from build123d import *

# Parameters (mm, degrees)
SKETCH1_W                    = 79.375
SKETCH1_H                    = 660.4
BASE_FLANGE1_DEPTH           = 3.175
EDGE_FLANGE1_STRIP_W         = 19.05
EDGE_FLANGE1_STRIP_H         = 3.175
EDGE_FLANGE1_STRIP_CUT_DEPTH = 660.4
EDGE_FLANGE1_DEPTH           = 660.4
EDGE_FLANGE3_STRIP_W         = 19.05
EDGE_FLANGE3_STRIP_H         = 3.175
EDGE_FLANGE3_STRIP_CUT_DEPTH = 660.4
EDGE_FLANGE3_DEPTH           = 660.4
SKETCH21_R                   = 2.45745
CUT_EXTRUDE2_DEPTH           = 703.314018976
SKETCH24_R                   = 2.45745
CUT_EXTRUDE3_DEPTH           = 3.175
SKETCH25_R                   = 4.3688
SKETCH25_R_2                 = 2.45745
CUT_EXTRUDE4_DEPTH           = 3.175
EDGE_FLANGE4_START           = -3.175
EDGE_FLANGE4_DEPTH           = 225.425
EDGE_FLANGE4_2_DEPTH         = 6.35
EDGE_FLANGE4_START_2         = 215.9
EDGE_FLANGE4_3_DEPTH         = 6.35
EDGE_FLANGE4_START_3         = 3.175
EDGE_FLANGE4_4_DEPTH         = 212.725
EDGE_FLANGE5_START           = -3.175
EDGE_FLANGE5_DEPTH           = 225.425
EDGE_FLANGE5_2_DEPTH         = 6.35
EDGE_FLANGE5_START_2         = 215.9
EDGE_FLANGE5_3_DEPTH         = 6.35
EDGE_FLANGE5_START_3         = 3.175
EDGE_FLANGE5_4_DEPTH         = 212.725
SKETCH32_R                   = 2.45745
CUT_EXTRUDE5_DEPTH           = 702.301371113
FILLET1_R                    = 3.175


# Read off the part's stored shape, not the designer's step: Edge-Flange4, Edge-Flange5
# Sheet-metal steps are written as plain solids
with BuildPart() as part:
    # Sketch1 → Base-Flange1 (new body)
    with BuildSketch(Plane(origin=(0, 0, 0), x_dir=(0, 0, -1), z_dir=(1, 0, 0))):
        with Locations((39.6875, 330.2)):
            Rectangle(SKETCH1_W, SKETCH1_H)
    extrude(amount=-BASE_FLANGE1_DEPTH)

    # Edge-Flange1 strip (across the edge) → Edge-Flange1 strip cut (cut)
    with BuildSketch(Plane(origin=(0, 0, -79.375), x_dir=(0, 0, 1), z_dir=(0, 1, 0))):
        with Locations((-3.175, -1.5875)):
            Rectangle(EDGE_FLANGE1_STRIP_W, EDGE_FLANGE1_STRIP_H)
    extrude(amount=EDGE_FLANGE1_STRIP_CUT_DEPTH, mode=Mode.SUBTRACT)

    # Edge-Flange1 section (across the edge) → Edge-Flange1 (add)
    with BuildSketch(Plane(origin=(0, 0, -79.375), x_dir=(0, 0, 1), z_dir=(0, 1, 0))):
        with BuildLine():
            Line((0, 3.175), (0, 222.25))
            Line((0, 222.25), (3.175, 222.25))
            Line((3.175, 222.25), (3.175, 3.175))
            ThreePointArc((3.175, 3.175), (4.10493597, 0.92993597), (6.35, 0))
            Line((6.35, 0), (6.35, -3.175))
            ThreePointArc((6.35, -3.175), (1.859871939, -1.315128061), (0, 3.175))
        make_face()
    extrude(amount=EDGE_FLANGE1_DEPTH)

    # Edge-Flange3 strip (across the edge) → Edge-Flange3 strip cut (cut)
    with BuildSketch(Plane(origin=(222.25, 0, -76.2), x_dir=(-1, 0, 0), z_dir=(0, 1, 0))):
        with Locations((-3.175, -1.5875)):
            Rectangle(EDGE_FLANGE3_STRIP_W, EDGE_FLANGE3_STRIP_H)
    extrude(amount=EDGE_FLANGE3_STRIP_CUT_DEPTH, mode=Mode.SUBTRACT)

    # Edge-Flange3 section (across the edge) → Edge-Flange3 (add)
    with BuildSketch(Plane(origin=(222.25, 0, -76.2), x_dir=(-1, 0, 0), z_dir=(0, 1, 0))):
        with BuildLine():
            Line((0, 3.175), (0, 28.575))
            Line((0, 28.575), (3.175, 28.575))
            Line((3.175, 28.575), (3.175, 3.175))
            ThreePointArc((3.175, 3.175), (4.10493597, 0.92993597), (6.35, 0))
            Line((6.35, 0), (6.35, -3.175))
            ThreePointArc((6.35, -3.175), (1.859871939, -1.315128061), (0, 3.175))
        make_face()
    extrude(amount=EDGE_FLANGE3_DEPTH)

    # Sketch21 → Cut-Extrude2 (cut, through all)
    with BuildSketch(Plane.ZY.offset(3.175)):
        with Locations((-12.7, 647.7)):
            Circle(SKETCH21_R)
        with Locations((-12.7, 436.118)):
            Circle(SKETCH21_R)
        with Locations((-12.7, 224.536)):
            Circle(SKETCH21_R)
        with Locations((-12.7, 12.954)):
            Circle(SKETCH21_R)
    extrude(amount=-CUT_EXTRUDE2_DEPTH, mode=Mode.SUBTRACT)

    # Sketch24 → Cut-Extrude3 (cut)
    with BuildSketch(Plane(origin=(222.25, 0, 0), x_dir=(0, 0, -1), z_dir=(1, 0, 0))):
        with Locations((60.325, 647.7)):
            Circle(SKETCH24_R)
        with Locations((60.325, 436.118)):
            Circle(SKETCH24_R)
        with Locations((60.325, 224.536)):
            Circle(SKETCH24_R)
        with Locations((60.325, 12.954)):
            Circle(SKETCH24_R)
    extrude(amount=-CUT_EXTRUDE3_DEPTH, mode=Mode.SUBTRACT)

    # Sketch25 → Cut-Extrude4 (cut)
    with BuildSketch(Plane(origin=(0, 0, -79.375), x_dir=(-1, 0, 0), z_dir=(0, 0, -1))):
        with Locations((-203.2, 590.55)):
            Circle(SKETCH25_R)
        with Locations((-19.05, 590.55)):
            Circle(SKETCH25_R)
        with Locations((-19.05, 330.2)):
            Circle(SKETCH25_R)
        with Locations((-203.2, 330.2)):
            Circle(SKETCH25_R)
        with Locations((-19.05, 561.975)):
            Circle(SKETCH25_R_2)
        with Locations((-203.2, 561.975)):
            Circle(SKETCH25_R_2)
        with Locations((-203.2, 355.6)):
            Circle(SKETCH25_R_2)
        with Locations((-19.05, 355.6)):
            Circle(SKETCH25_R_2)
        with Locations(Location((-203.2, 304.8, 0), (0, 0, 180))):
            Circle(SKETCH25_R_2)
        with Locations(Location((-19.05, 304.8, 0), (0, 0, 180))):
            Circle(SKETCH25_R_2)
        with Locations(Location((-19.05, 98.425, 0), (0, 0, 180))):
            Circle(SKETCH25_R_2)
        with Locations(Location((-203.2, 98.425, 0), (0, 0, 180))):
            Circle(SKETCH25_R_2)
        with Locations((-203.2, 69.85)):
            Circle(SKETCH25_R)
        with Locations((-19.05, 69.85)):
            Circle(SKETCH25_R)
    extrude(amount=-CUT_EXTRUDE4_DEPTH, mode=Mode.SUBTRACT)

    # Edge-Flange4 outline → Edge-Flange4 (cut)
    with BuildSketch(Plane.YZ.offset(EDGE_FLANGE4_START)):
        with BuildLine():
            ThreePointArc((660.4, -73.025), (658.540128061, -77.515128061), (654.05, -79.375))
            Line((654.05, -79.375), (660.4, -79.375))
            Line((660.4, -79.375), (660.4, -73.025))
        make_face()
        with BuildLine():
            ThreePointArc((654.05, -76.2), (656.29506403, -75.27006403), (657.225, -73.025))
            Line((657.225, -73.025), (654.05, -73.025))
            Line((654.05, -73.025), (654.05, -76.2))
        make_face()
    extrude(amount=EDGE_FLANGE4_DEPTH, mode=Mode.SUBTRACT)

    # Edge-Flange4 2 outline → Edge-Flange4 2 (cut)
    with BuildSketch(Plane.YZ.offset(EDGE_FLANGE4_START)):
        with BuildLine():
            Line((660.4, -73.025), (657.225, -73.025))
            ThreePointArc((657.225, -73.025), (656.29506403, -75.27006403), (654.05, -76.2))
            Line((654.05, -76.2), (654.05, -79.375))
            ThreePointArc((654.05, -79.375), (658.540128061, -77.515128061), (660.4, -73.025))
        make_face()
    extrude(amount=EDGE_FLANGE4_2_DEPTH, mode=Mode.SUBTRACT)

    # Edge-Flange4 3 outline → Edge-Flange4 3 (cut)
    with BuildSketch(Plane.YZ.offset(EDGE_FLANGE4_START_2)):
        with BuildLine():
            Line((660.4, -73.025), (657.225, -73.025))
            ThreePointArc((657.225, -73.025), (656.29506403, -75.27006403), (654.05, -76.2))
            Line((654.05, -76.2), (654.05, -79.375))
            ThreePointArc((654.05, -79.375), (658.540128061, -77.515128061), (660.4, -73.025))
        make_face()
    extrude(amount=EDGE_FLANGE4_3_DEPTH, mode=Mode.SUBTRACT)

    # Edge-Flange4 4 outline → Edge-Flange4 4 (add)
    with BuildSketch(Plane.YZ.offset(EDGE_FLANGE4_START_3)):
        with BuildLine():
            ThreePointArc((659.549261315, -76.2), (660.183628997, -74.668500936), (660.4, -73.025))
            Line((660.4, -73.025), (660.4, -47.625))
            Line((660.4, -47.625), (657.225, -47.625))
            Line((657.225, -47.625), (657.225, -73.025))
            ThreePointArc((657.225, -73.025), (656.29506403, -75.27006403), (654.05, -76.2))
            Line((654.05, -76.2), (659.549261315, -76.2))
        make_face()
    extrude(amount=EDGE_FLANGE4_4_DEPTH)

    # Edge-Flange5 outline → Edge-Flange5 (cut)
    with BuildSketch(Plane.YZ.offset(EDGE_FLANGE5_START)):
        with BuildLine():
            Line((0, -73.025), (0, -79.375))
            Line((0, -79.375), (6.35, -79.375))
            ThreePointArc((6.35, -79.375), (1.859871939, -77.515128061), (0, -73.025))
        make_face()
        with BuildLine():
            Line((6.35, -73.025), (3.175, -73.025))
            ThreePointArc((3.175, -73.025), (4.10493597, -75.27006403), (6.35, -76.2))
            Line((6.35, -76.2), (6.35, -73.025))
        make_face()
    extrude(amount=EDGE_FLANGE5_DEPTH, mode=Mode.SUBTRACT)

    # Edge-Flange5 2 outline → Edge-Flange5 2 (cut)
    with BuildSketch(Plane.YZ.offset(EDGE_FLANGE5_START)):
        with BuildLine():
            Line((3.175, -73.025), (0, -73.025))
            ThreePointArc((0, -73.025), (1.859871939, -77.515128061), (6.35, -79.375))
            Line((6.35, -79.375), (6.35, -76.2))
            ThreePointArc((6.35, -76.2), (4.10493597, -75.27006403), (3.175, -73.025))
        make_face()
    extrude(amount=EDGE_FLANGE5_2_DEPTH, mode=Mode.SUBTRACT)

    # Edge-Flange5 3 outline → Edge-Flange5 3 (cut)
    with BuildSketch(Plane.YZ.offset(EDGE_FLANGE5_START_2)):
        with BuildLine():
            Line((3.175, -73.025), (0, -73.025))
            ThreePointArc((0, -73.025), (1.859871939, -77.515128061), (6.35, -79.375))
            Line((6.35, -79.375), (6.35, -76.2))
            ThreePointArc((6.35, -76.2), (4.10493597, -75.27006403), (3.175, -73.025))
        make_face()
    extrude(amount=EDGE_FLANGE5_3_DEPTH, mode=Mode.SUBTRACT)

    # Edge-Flange5 4 outline → Edge-Flange5 4 (add)
    with BuildSketch(Plane.YZ.offset(EDGE_FLANGE5_START_3)):
        with BuildLine():
            Line((0, -47.625), (0, -73.025))
            ThreePointArc((0, -73.025), (0.216371003, -74.668500936), (0.850738685, -76.2))
            Line((0.850738685, -76.2), (6.35, -76.2))
            ThreePointArc((6.35, -76.2), (4.10493597, -75.27006403), (3.175, -73.025))
            Line((3.175, -73.025), (3.175, -47.625))
            Line((3.175, -47.625), (0, -47.625))
        make_face()
    extrude(amount=EDGE_FLANGE5_4_DEPTH)

    # Sketch32 → Cut-Extrude5 (cut, through all)
    with BuildSketch(Plane.XZ):
        with Locations(Location((25.4, -60.325, 0), (0, 0, 270))):
            Circle(SKETCH32_R)
        with Locations(Location((196.85, -60.325, 0), (0, 0, 270))):
            Circle(SKETCH32_R)
    extrude(amount=-CUT_EXTRUDE5_DEPTH, mode=Mode.SUBTRACT)

    # Fillet1
    fillet1_edges = [part.edges().sort_by_distance(p)[0] for p in [
        (220.6625, 0, -47.625),
        (215.9, 1.5875, -47.625),
        (220.6625, 0, -73.025),
        (-1.5875, 0, 0),
        (3.175, 1.5875, -47.625),
        (-1.5875, 0, -73.025),
        (-1.5875, 660.4, -73.025),
        (-1.5875, 660.4, 0),
        (3.175, 658.8125, -47.625),
        (220.6625, 660.4, -73.025),
        (215.9, 658.8125, -47.625),
        (220.6625, 660.4, -47.625),
    ]]
    fillet(fillet1_edges, radius=FILLET1_R)


solid = part.part
Read the model definition and answer for the solid it produces. Units are mm, in the model's axes. A direction names the side the tool comes from. Round coordinates to 2 decimals unless told otherwise and drop trailing zeros. Order: outer loops, then holes, each group sorted by start corner. A loop starts at its lowest first (then second) coordinate and runs counter-clockwise, first axis right, second up. Notation, with made-up numbers: (76.25, 61.5) - (92.25, 61.5) arc R20 cw to (92.25, 87.5) - close; hole circle Ø4 at (63, 44.5). An arc over 180 degrees is marked (long way). Use one line per item in the form item = value. Start each with the question number.
(1) For faces 4 (the face through (0, 335, -36)), 5 (the face through (108, 657.225, -60)), 6 (the face through (108, 660.4, -61)), determine the directions among +Z, -Z, +X, -X, +Y, -Y from which every point of the face is accessible in a straight line to the end or side of a thin tool.
(2) The part is cut by section C-C (z = -31). Give the vertices of the cut face in (x, y) (3 decimals), then the cut area to 3 significant figures.
(3) The part is cut by section B-B (y = 192). Give the vertices of the cut face in (x, z) (3 decimals).
(4) Find the intervals of material crossed by line 1 along Y through (x, z) = (-0.8, -12.7); line 2 along X through (y, z) = (355, -78); line 3 along X through (y, z) = (465.5, -65) (3 decimals), in increasing order. Write a range as from..to.
(5) Determine the mould class of faces 1 (the face through (219.075, 326, -60)), 2 (the face through (108, 326, -79.375)), 3 (the face through (-3.175, 335, -36)) for opening direction X: +X half, -X half, draft (parallel to the pull), parting line (faces both ways), or undercut.
(6) The part is cut by section A-A (x = 73.5). Give the vertices of the cut face in (y, z) (3 decimals), then the cut area to 3 significant figures.
(7) Flat-ended cylindrical pins translate along their axes: pin 1 Ø5.5 at (y, z) = (647.7, -12.7) entering from +X; pin 2 Ø11.5 at (x, y) = (19.05, 69.85) entering from +Z; pin 3 Ø1.9 at (x, z) = (1, -77.5) entering from -Y; pin 4 Ø5 at (x, y) = (203.2, 69.85) entering from +Z. Find the tip coordinate at first contact, or state that the pin passes through.
Checked values:
q1.face_4 = +Z, +Y, -Y
q1.face_5 = +Z
q1.face_6 = +Z, -Z, +X, -X, +Y
q2.outline = (-3.175, 0) - (0, 0) - (0, 660.4) - (-3.175, 660.4) - close
q2.area = 2,100 mm^2
q3.outline = (-3.175, -73.025) arc R6.35 ccw to (3.175, -79.375) - (215.9, -79.375) arc R6.35 ccw to (222.25, -73.025) - (222.25, -47.625) - (219.075, -47.625) - (219.075, -73.025) arc R3.175 cw to (215.9, -76.2) - (3.175, -76.2) arc R3.175 cw to (0, -73.025) - (0, 0) - (-3.175, 0) - close
q4.line_1 = 0..10.5, 15.41..222.08, 226.99..433.66, 438.58..645.24, 650.16..660.4
q4.line_2 = -0.77..16.67, 21.43..200.82, 205.58..219.85
q4.line_3 = -3.175..0, 219.075..222.25
q5.face_1 = undercut
q5.face_2 = draft
q5.face_3 = -X half
q6.outline = (0, -73.025) arc R6.35 ccw to (6.35, -79.375) - (654.05, -79.375) arc R6.35 ccw to (660.4, -73.025) - (660.4, -47.625) - (657.225, -47.625) - (657.225, -73.025) arc R3.175 cw to (654.05, -76.2) - (6.35, -76.2) arc R3.175 cw to (3.175, -73.025) - (3.175, -47.625) - (0, -47.625) - close
q6.area = 2,270 mm^2
q7.pin_1 = 0
q7.pin_2 = -76.2
q7.pin_3 = 6.35
q7.pin_4 = through
